```python
from build123d import *

# Parameters (mm, degrees)
F0_W     = 54
F0_H     = 54
F1_DEPTH = 867
F2_R     = 7
F3_DEPTH = 3
F4_W     = 60
F4_H     = 60
F4_R     = 6
F5_DEPTH = 6
F7_R     = 6
F8_DEPTH = 70


# Not quite as in the source:
# - a feature names something its author has since deleted; it is built from what else it names


with BuildPart() as f1:
    # F0 (on Front) → F1 (new body)
    with BuildSketch(Plane.XZ):
        with BuildLine():
            ThreePointArc((-28.9867345989, -60.995567819), (-30.4512006929, -57.460033913), (-33.9867345989, -55.995567819))
            Line((-33.9867345989, -55.995567819), (-83.9867345989, -55.995567819))
            ThreePointArc((-83.9867345989, -55.995567819), (-87.5222685048, -57.460033913), (-88.9867345989, -60.995567819))
            Line((-88.9867345989, -60.995567819), (-88.9867345989, -110.995567819))
            ThreePointArc((-88.9867345989, -110.995567819), (-87.5222685048, -114.5311017249), (-83.9867345989, -115.995567819))
            Line((-83.9867345989, -115.995567819), (-33.9867345989, -115.995567819))
            ThreePointArc((-33.9867345989, -115.995567819), (-30.4512006929, -114.5311017249), (-28.9867345989, -110.995567819))
            Line((-28.9867345989, -110.995567819), (-28.9867345989, -60.995567819))
        make_face()
        with Locations((-58.9867345989, -85.995567819)):
            Rectangle(F0_W, F0_H, mode=Mode.SUBTRACT)
    extrude(amount=-F1_DEPTH)

    # F2 (on face) → F3 (cut, through all)
    with BuildSketch(Plane.YZ.offset(-28.9867345989)):
        with Locations((20, -85.995567819)):
            Circle(F2_R)
        with Locations((50, -85.995567819)):
            Circle(F2_R)
    extrude(amount=-F3_DEPTH, mode=Mode.SUBTRACT)

    # F4 (on face) → F5 (join)
    with BuildSketch(Plane(origin=(0, 867, 0), x_dir=(-1, 0, 0), z_dir=(0, 1, 0))):
        with Locations((58.9867345989, -85.995567819)):
            Rectangle(F4_W, F4_H)
        with Locations((58.9867345989, -85.995567819)):
            Circle(F4_R, mode=Mode.SUBTRACT)
    extrude(amount=F5_DEPTH)

    # F7 (on offset) → F8 (join)
    with BuildSketch(Plane(origin=(0, 867, 0), x_dir=(-1, 0, 0), z_dir=(0, 1, 0))):
        with Locations((58.9867345989, -85.995567819)):
            Circle(F7_R)
    extrude(amount=F8_DEPTH)


solid = f1.part
```
The listing builds one solid part. Answer for the finished solid, in the listing's coordinates (mm). A direction names the side the tool comes from. Give positions to 0.01 mm unless a question says otherwise; leave off trailing zeros. Order: outer loops, then holes, each group sorted by start corner. A loop starts at its lowest first (then second) coordinate and runs counter-clockwise, first axis right, second up. Notation, with made-up numbers: (-14, 31.5) - (5, 31.5) arc R11 cw to (5, 36.5) - close; hole circle Ø4 at (18, 81). An arc over 180 degrees is marked (long way). Answer in a Markdown table with one row per item. Add a question column.
Q1. Find the intervals of material crossed by line 1 along X through (y, z) = (844.5, -85.5); line 2 along Z through (x, y) = (-42.5, 125); line 3 along Y through (x, z) = (-62, -99), in increasing order. Write a range as [from, to].
Q2. The part is cut by section B-B (z = -71). Determine the outline of the cut face in (x, y), then the cut area to 3 significant figures.
Q3. The part is cut by section A-A (y = 596.5). Determine the outline of the cut face in (x, z).
Q4. Which of the six approach directions +Z, -Z, +X, -X, +Y, -Y give full straight-line access (tool end or side, diameter ignored) to faces 1 (the flat face through (-59, 430, -115.996)), 2 (the flat face through (-59, 867, -86))?
Q5. For a pull along X with two mould halves and no side action, classify faces 3 (the flat face through (-85.987, 427, -86)), 4 (the flat face through (-59, 0, -57)), 5 (the flat face through (-88.987, 430, -86)) as released by +X, released by -X, zero draft, split by the parting line, or undercut.
Q6. Given P1, Ø10, axis at x = -38.5, z = -71, coming from the -Y side; P2, Ø4, axis at x = -31.5, z = -58, coming from the -Y side; P3, Ø8.5, axis at y = 20, z = -86, coming from the +X side; P4, Ø1.5, axis at x = -79.5, z = -101.5, coming from the +Y side, each flat-ended and moving along its own axis, determine where each tip first touches the part or whether it passes through.
Determined:
| question | item | result |
|---|---|---|
| 1 | line 1 | x = [-88.99, -85.99], [-31.99, -28.99] |
| 1 | line 2 | z = [-116, -113], [-59, -56] |
| 1 | line 3 | y = [867, 873] |
| 2 | outline | (-88.99, 0) - (-85.99, 0) - (-85.99, 867) - (-31.99, 867) - (-31.99, 0) - (-28.99, 0) - (-28.99, 873) - (-88.99, 873) - close |
| 2 | area | 5,560 mm² |
| 3 | outline | (-88.99, -111) arc R5 ccw to (-83.99, -116) - (-33.99, -116) arc R5 ccw to (-28.99, -111) - (-28.99, -61) arc R5 ccw to (-33.99, -56) - (-83.99, -56) arc R5 ccw to (-88.99, -61) - close; hole (-85.99, -113) - (-31.99, -113) - (-31.99, -59) - (-85.99, -59) - close |
| 4 | face 1 | -Z, +X, -X, +Y, -Y |
| 4 | face 2 | -Y |
| 5 | face 3 | undercut |
| 5 | face 4 | zero draft |
| 5 | face 5 | released by -X |
| 6 | P1 | stops at y = 867 |
| 6 | P2 | stops at y = 0 |
| 6 | P3 | stops at x = -85.99 |
| 6 | P4 | stops at y = 873 |
